Job drawing, mm, ordinate dimensions from the low corner. One solid piece. A direction names the side the tool comes from. Round coordinates to 2 decimals unless told otherwise and drop trailing zeros. Order: outer loops, then holes, each group sorted by start corner. A loop starts at its lowest first (then second) coordinate and runs counter-clockwise, first axis right, second up. Notation, with made-up numbers: M 6,22.5 L 16,22.5 A29 ccw 16,56.5 Z; hole C -28.5,-32 d2. An arc over 180 degrees is marked long. Answer as a JSON object with one key per item and string values. Group by question number.
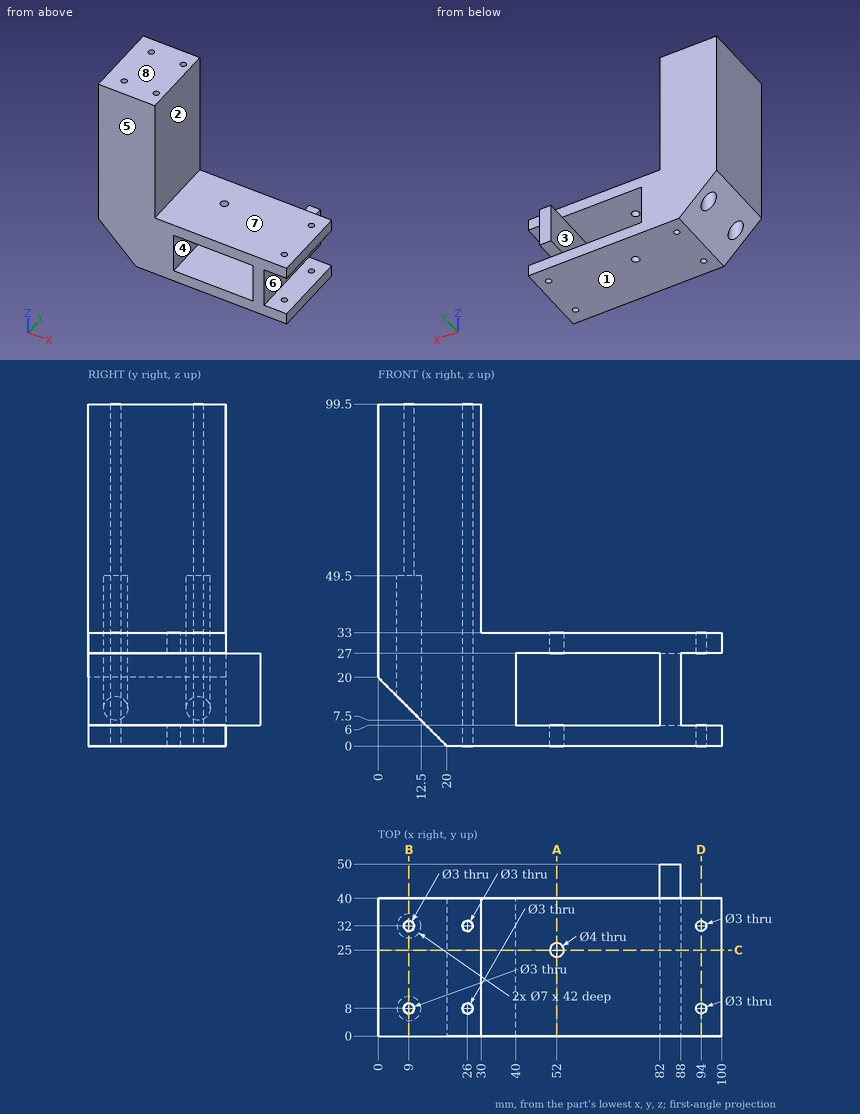
Item 1: Flat gauge pins, fed straight in: pin 1 Ø8 at (x, y) = (85, 35) entering from +Z; pin 2 Ø3 at (y, z) = (31.5, 17) entering from -X; pin 3 Ø6 at (x, z) = (34.5, 27.5) entering from +Y; pin 4 Ø1.8 at (x, y) = (9, 32) entering from +Z. Where does each tip first touch, or does it go through?
Item 2: Cut at A-A, the plane x = 52. Give the cut face in (y, z), and give its area (3 significant figures).
Item 3: Cut at C-C, the plane y = 25. Give the cut face in (x, z).
Item 4: Two-plate mould, pull along Z, no slides. Class the marked faces 1, 2 and 3: +Z half, -Z half, draft (parallel to the pull), parting line (faces both ways), or undercut.
Item 5: Cut at B-B, the plane x = 9. Give the cut face in (y, z), and give its area (3 significant figures).
Item 6: 3-axis set-ups, long thin cutter, end or side, ignore diameter. For the marked faces 4, 5, 6, 7 and 8: which of +Z, -Z, +X, -X, +Y, -Y reach the whole face in a straight line?
Item 7: Cut at D-D, the plane x = 94. Give the cut face in (y, z).
Item 8: Drill centre lines: line 1 (X direction, y = 32, z = 74); line 2 (Y direction, x = 9, z = 21); line 3 (Y direction, x = 9, z = 89). Where is each one in solid material? Low to high. Write a range as [from, to].
Response values:
{
 "1": {"pin 1": "z = 33", "pin 2": "x = 1.5", "pin 3": "y = 40", "pin 4": "through"},
 "2": {"outline": "M 0,0 L 23,0 L 23,6 L 0,6 Z; M 0,27 L 23,27 L 23,33 L 0,33 Z; M 27,0 L 40,0 L 40,6 L 27,6 Z; M 27,27 L 40,27 L 40,33 L 27,33 Z", "area": "432 mm^2"},
 "3": {"outline": "M 0,20 L 20,0 L 50,0 L 50,6 L 40,6 L 40,27 L 50,27 L 50,33 L 30,33 L 30,99.5 L 0,99.5 Z; M 54,0 L 100,0 L 100,6 L 88,6 L 88,27 L 100,27 L 100,33 L 54,33 L 54,27 L 82,27 L 82,6 L 54,6 Z"},
 "4": {"face 1": "-Z half", "face 2": "draft", "face 3": "undercut"},
 "5": {"outline": "M 0,11 L 4.5,11 L 4.5,49.5 L 6.5,49.5 L 6.5,99.5 L 0,99.5 Z; M 9.5,49.5 L 11.5,49.5 L 11.5,11 L 28.5,11 L 28.5,49.5 L 30.5,49.5 L 30.5,99.5 L 9.5,99.5 Z; M 33.5,49.5 L 35.5,49.5 L 35.5,11 L 40,11 L 40,99.5 L 33.5,99.5 Z", "area": "2,700 mm^2"},
 "6": {"face 4": "+Y, -Y", "face 5": "+Z, -Z, +X, -X, -Y", "face 6": "+X, +Y, -Y", "face 7": "+Z, +X, +Y, -Y", "face 8": "+Z, +X, -X, +Y, -Y"},
 "7": {"outline": "M 0,0 L 6.5,0 L 6.5,6 L 0,6 Z; M 0,27 L 6.5,27 L 6.5,33 L 0,33 Z; M 9.5,0 L 30.5,0 L 30.5,6 L 9.5,6 Z; M 9.5,27 L 30.5,27 L 30.5,33 L 9.5,33 Z; M 33.5,0 L 40,0 L 40,6 L 33.5,6 Z; M 33.5,27 L 40,27 L 40,33 L 33.5,33 Z"},
 "8": {"line 1": "[0, 7.5], [10.5, 24.5], [27.5, 30]", "line 2": "[0, 4.5], [11.5, 28.5], [35.5, 40]", "line 3": "[0, 6.5], [9.5, 30.5], [33.5, 40]"}
}
